from build123d import *

# Parameters (mm, degrees)
IZIM1_W                     = 500
IZIM1_H                     = 500
Y_KSEKLIK_EKSTR_ZYON1_DEPTH = 100
IZIM2_W                     = 100
IZIM2_H                     = 200
Y_KSEKLIK_EKSTR_ZYON2_DEPTH = 200
IZIM3_R                     = 50
Y_KSEKLIK_EKSTR_ZYON3_DEPTH = 50
IZIM4_R                     = 30
Y_KSEKLIK_EKSTR_ZYON4_DEPTH = 50


with BuildPart() as part:
    # Çizim1 → Yükseklik-Ekstrüzyon1 (new body)
    with BuildSketch(Plane(origin=(0, 0, 0), x_dir=(1, 0, 0), z_dir=(0, 1, 0))):
        Rectangle(IZIM1_W, IZIM1_H)
    extrude(amount=Y_KSEKLIK_EKSTR_ZYON1_DEPTH)

    # Çizim2 → Yükseklik-Ekstrüzyon2 (add)
    with BuildSketch(Plane(origin=(0, 100, 0), x_dir=(1, 0, 0), z_dir=(0, 1, 0))):
        with Locations((-50, 0)):
            Rectangle(IZIM2_W, IZIM2_H)
    extrude(amount=Y_KSEKLIK_EKSTR_ZYON2_DEPTH)

    # Çizim3 → Yükseklik-Ekstrüzyon3 (add)
    with BuildSketch(Plane(origin=(0, 0, 0), x_dir=(0, 0, -1), z_dir=(1, 0, 0))):
        with Locations(Location((0, 200, 0), (0, 0, 180))):
            Circle(IZIM3_R)
    extrude(amount=Y_KSEKLIK_EKSTR_ZYON3_DEPTH)

    # Çizim4 → Yükseklik-Ekstrüzyon4 (add)
    with BuildSketch(Plane(origin=(50, 0, 0), x_dir=(0, 0, -1), z_dir=(1, 0, 0))):
        with Locations((0, 200)):
            Circle(IZIM4_R)
    extrude(amount=Y_KSEKLIK_EKSTR_ZYON4_DEPTH)


solid = part.part
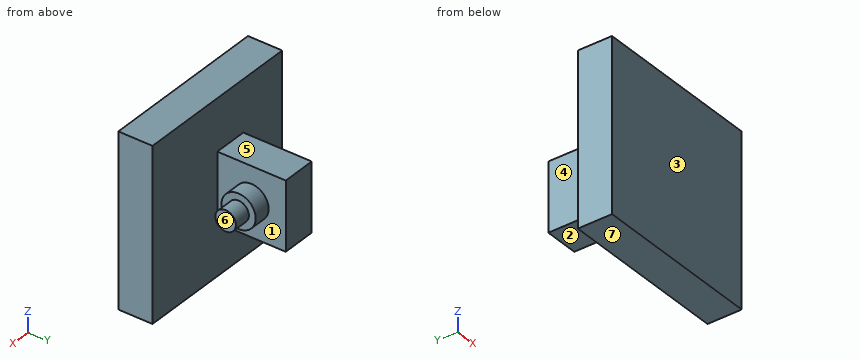
The model under review builds one solid part; all positions refer to its coordinate system, in mm. Face numbers are marked on the shaded views. A direction names the side the tool comes from. Give positions to 0.01 mm unless a question says otherwise; leave off trailing zeros. Write each loop counter-clockwise with the first axis right and the second up, starting at its lowest first coordinate (ties: lowest second). Pieces come first, ordered by that corner, then holes. Notation, with made-up numbers: M 17,84.5 L 43,84.5 A31 ccw 43,108.5 Z; hole C 78.5,39 d1. An arc over 180 degrees is marked long. One line per question, with ' | ' between items. Start each with the question number.
Item 1: We need section C-C on z = 0. Write out the cut boundary in (x, y).
Item 2: Wall thickness on line 1 (Y direction, x = 163, z = 80.5); line 2 (Y direction, x = 88.5, z = -3); line 3 (X direction, y = 217.5, z = 88.5): over which ranges is each line inside the solid? List them lowest first. Write a range as from..to.
Item 3: We need section B-B on x = 75. Write out the cut boundary in (y, z), plus the area to 3 significant figures.
Item 4: For the marked faces 4, 5, 6 and 7, list the 3-axis set-ups (+Z, -Z, +X, -X, +Y, -Y) from which the entire face can be reached by the end or side of a thin tool; tool diameter is ignored.
Item 5: Draft analysis for pull direction Y (two halves, no side actions). For the marked faces 1, 2 and 3, state which applies: released by +Y, released by -Y, zero draft, split by the parting line, or undercut.
Item 6: We need section A-A on x = -55.5. Write out the cut boundary in (y, z).
Item 7: For pin 1 (8 mm diameter, centred on x = -77.5, y = 244.5, fed in from -Z); pin 2 (10 mm diameter, centred on y = 256.5, z = 3, fed in from +X); pin 3 (8 mm diameter, centred on x = -54, z = -146, fed in from +Y), all flat-tipped, find the tip position at first contact; note any pin that passes through.
Item 8: We need section D-D on y = 200. Write out the cut boundary in (x, z), plus the area to 3 significant figures.
Results found:
1) outline: M -250,0 L 250,0 L 250,100 L 0,100 L 0,150 L 50,150 L 50,170 L 100,170 L 100,230 L 50,230 L 50,250 L 0,250 L 0,300 L -100,300 L -100,100 L -250,100 Z
2) line 1: y = 0..100 | line 2: y = 0..100, 170.15..229.85 | line 3: x = -100..0
3) outline: M 0,-250 L 100,-250 L 100,250 L 0,250 Z; C 200,0 d60 | area: 52,800 mm2
4) face 4: +Z, -Z, -X, +Y | face 5: +Z, +X, -X, +Y | face 6: +Z, -Z, +X, +Y | face 7: -Z, +X, -X, +Y, -Y
5) face 1: undercut | face 2: zero draft | face 3: released by -Y
6) outline: M 0,-250 L 100,-250 L 100,-100 L 300,-100 L 300,100 L 100,100 L 100,250 L 0,250 Z
7) pin 1: stops at z = -100 | pin 2: stops at x = 0 | pin 3: stops at y = 100
8) outline: M -100,-100 L 0,-100 L 0,-50 L 50,-50 L 50,-30 L 100,-30 L 100,30 L 50,30 L 50,50 L 0,50 L 0,100 L -100,100 Z | area: 28,000 mm2
